```python
from build123d import *

# Parameters (mm, degrees)
SKETCH_1_W               = 60
SKETCH_1_H               = 30
EXTRUDE_1_DEPTH          = 3
SKETCH_2_R               = 1.5
CUT_EXTRUDE_1_DEPTH      = 3
MIRROR_2_COPY_1_SKETCH_R = 1.5
MIRROR_2_COPY_1_DEPTH    = 3
FILLET_2_R               = 2
SKETCH_5_R               = 6
EXTRUDE_2_DEPTH          = 30
SKETCH_6_W               = 12
SKETCH_6_H               = 5
EXTRUDE_3_DEPTH          = 30
SKETCH_7_R               = 4
CUT_EXTRUDE_4_DEPTH      = 31
SKETCH_8_W               = 8
SKETCH_8_H               = 9.1545719
EXTRUDE_4_DEPTH          = 30
SKETCH_9_W               = 2.976845738
SKETCH_9_H               = 12.85930144
CUT_EXTRUDE_5_DEPTH      = 31
SKETCH_10_R              = 1.5
CUT_EXTRUDE_6_DEPTH      = 35


with BuildPart() as part:
    # 草图1 → 凸台-拉伸1 (new body)
    with BuildSketch(Plane(origin=(0, 0, 0), x_dir=(1, 0, 0), z_dir=(0, 1, 0))):
        Rectangle(SKETCH_1_W, SKETCH_1_H)
    extrude(amount=EXTRUDE_1_DEPTH)

    # 草图2 → 切除-拉伸1 (cut)
    with BuildSketch(Plane(origin=(0, 3, 0), x_dir=(1, 0, 0), z_dir=(0, 1, 0))):
        with Locations((-24, -9)):
            Circle(SKETCH_2_R)
    cut_extrude_1 = extrude(amount=-CUT_EXTRUDE_1_DEPTH, mode=Mode.SUBTRACT)

    # 镜向1: 切除-拉伸1 across plane
    add(cut_extrude_1.mirror(Plane.XY), mode=Mode.SUBTRACT)

    # 镜向2: 切除-拉伸1 across plane
    add(cut_extrude_1.mirror(Plane(origin=(0, 0, 0), x_dir=(0, 0, 1), z_dir=(1, 0, 0))), mode=Mode.SUBTRACT)

    # 镜向2 copy 1 sketch → 镜向2 copy 1 (cut)
    with BuildSketch(Plane(origin=(0, 3, 0), x_dir=(-1, 0, 0), z_dir=(0, 1, 0))):
        with Locations((-24, -9)):
            Circle(MIRROR_2_COPY_1_SKETCH_R)
    extrude(amount=-MIRROR_2_COPY_1_DEPTH, mode=Mode.SUBTRACT)

    # 圆角2
    fillet_2_edges = [part.edges().sort_by_distance(p)[0] for p in [
        (-30, 1.5, -15),
        (30, 1.5, -15),
        (30, 1.5, 15),
        (-30, 1.5, 15),
    ]]
    fillet(fillet_2_edges, radius=FILLET_2_R)

    # 草图5 → 凸台-拉伸2 (add)
    with BuildSketch(Plane.XY.offset(15)):
        with Locations((0, 8)):
            Circle(SKETCH_5_R)
    extrude(amount=-EXTRUDE_2_DEPTH)

    # 草图6 → 凸台-拉伸3 (add)
    with BuildSketch(Plane.XY.offset(15)):
        with Locations((0, 5.5)):
            Rectangle(SKETCH_6_W, SKETCH_6_H)
    extrude(amount=-EXTRUDE_3_DEPTH)

    # 草图7 → 切除-拉伸4 (cut, through all)
    with BuildSketch(Plane.XY.offset(15)):
        with Locations((0, 8)):
            Circle(SKETCH_7_R)
    extrude(amount=-CUT_EXTRUDE_4_DEPTH, mode=Mode.SUBTRACT)

    # 草图8 → 凸台-拉伸4 (add)
    with BuildSketch(Plane.XY.offset(15)):
        with Locations((0, 16.818752798)):
            Rectangle(SKETCH_8_W, SKETCH_8_H)
    extrude(amount=-EXTRUDE_4_DEPTH)

    # 草图9 → 切除-拉伸5 (cut, through all)
    with BuildSketch(Plane.XY.offset(15)):
        with Locations((0, 16.396965649)):
            Rectangle(SKETCH_9_W, SKETCH_9_H)
    extrude(amount=-CUT_EXTRUDE_5_DEPTH, mode=Mode.SUBTRACT)

    # 草图10 → 切除-拉伸6 (cut, through all)
    with BuildSketch(Plane(origin=(4, 0, 0), x_dir=(0, 0, -1), z_dir=(1, 0, 0))):
        with Locations((10.28698243, 16.934087351)):
            Circle(SKETCH_10_R)
        with Locations((0.28698243, 16.934087351)):
            Circle(SKETCH_10_R)
        with Locations((-9.71301757, 16.934087351)):
            Circle(SKETCH_10_R)
    extrude(amount=-CUT_EXTRUDE_6_DEPTH, mode=Mode.SUBTRACT)


solid = part.part
```
Can you work these out from the model? Positions are in its coordinate system, mm. A direction names the side the tool comes from. Coordinates: 2 decimals unless noted, no trailing zeros. Order: outer loops, then holes, each group sorted by start corner. A loop starts at its lowest first (then second) coordinate and runs counter-clockwise, first axis right, second up.
1. If we section it at C-C (z = 4): Please give me the cut outline in (x, y), then the cut area to 3 significant figures.
2. If we section it at A-A (x = -24): Please give me the cut outline in (y, z), then the cut area to 3 significant figures.
3. If we section it at D-D (y = 16): Give the number of separate pieces and of enclosed holes in the cut face, then the cut area to 3 significant figures.
4. If we section it at B-B (y = 19): Please give me the cut outline in (x, z), then the cut area to 3 significant figures.
5. Thinking about a two-plate mould opening in Z: for faces 4 (the face through (-29.43, 1.52, 14.4)), 5 (the face through (25.2, 1.5, -9.9)), 6 (the face through (-5.463, 10.482, 0.21)), which applies, +Z half, -Z half, draft (parallel to the pull), parting line (faces both ways), or undercut?
6. I'm going to push flat-ended pins straight in: pin 1 (5.5 mm diameter, centred on y = 6.5, z = 6.5, fed in from +X); pin 2 (1.5 mm diameter, centred on y = 6.5, z = -4, fed in from -X); pin 3 (2.5 mm diameter, centred on y = 18, z = 7, fed in from -X). Where does each tip first touch, or does it pass through?
7. For faces 1 (the face through (4, 15, 0)), 2 (the face through (-2.73, 17, -8.79)), 3 (the face through (-6, 5, 0)), which set-ups out of +Z, -Z, +X, -X, +Y, -Y let a thin tool reach every point of the face, with its end or its side?
8. I need wall thicknesses on line 1 (Z direction, x = -24, y = 1.85); line 2 (X direction, y = 19.5, z = -0.75); line 3 (Y direction, x = 21.5, z = 10.5). Which ranges of each line are inside material? Lowest first, please.
Entries:
1. outline: (-30, 0) - (30, 0) - (30, 3) - (6, 3) - (6, 8) arc R6 ccw to (4, 12.47) - (4, 21.4) - (1.49, 21.4) - (1.49, 11.71) arc R4 cw (long way) to (-1.49, 11.71) - (-1.49, 21.4) - (-4, 21.4) - (-4, 12.47) arc R6 ccw to (-6, 8) - (-6, 3) - (-30, 3) - close
1. area: 281 mm2
2. outline: (0, -15) - (3, -15) - (3, -10.5) - (0, -10.5) - close; (0, -7.5) - (3, -7.5) - (3, 7.5) - (0, 7.5) - close; (0, 10.5) - (3, 10.5) - (3, 15) - (0, 15) - close
2. area: 72.0 mm2
3. separate pieces: 8
3. enclosed holes: 0
3. area: 115 mm2
4. outline: (-4, -15) - (-1.49, -15) - (-1.49, 15) - (-4, 15) - close; (1.49, -15) - (4, -15) - (4, 15) - (1.49, 15) - close
4. area: 151 mm2
5. face 4: +Z half
5. face 5: undercut
5. face 6: draft
6. pin 1: stops at x = 6
6. pin 2: stops at x = -6
6. pin 3: stops at x = -4
7. face 1: +Z, -Z, +X, +Y
7. face 2: +X, -X
7. face 3: +Z, -Z, -X, +Y
8. line 1: z = -15 to -10.5, -7.5 to 7.5, 10.5 to 15
8. line 2: x = -4 to -1.49, 1.49 to 4
8. line 3: y = 0 to 3
